For this review, take the finished solid that the model builds, in its own axes (mm). Coordinates: 2 decimals unless noted, no trailing zeros. Loops run counter-clockwise (first coordinate to the right, second up) from the corner with the lowest first, then second, coordinate; pieces in that order, holes last. Notation, with made-up numbers: (-10, -14) -> (41, -14) arc R31 ccw to (41, 24) -> close; hole circle Ø11 at (35, -23). An arc over 180 degrees is marked (long way). One line per item, written item: value.
from build123d import *

# Parameters (mm, degrees)
SALIENTE_EXTRUIR1_DEPTH = 0.25
CORTAR_EXTRUIR1_REACH   = 2.25
CROQUIS2_W              = 0.5
CROQUIS2_H              = 0.2


with BuildPart() as part:
    # Croquis1 → Saliente-Extruir1 (new body)
    with BuildSketch(Plane.XY):
        with BuildLine():
            Line((-0.5, -2.449489743), (-0.5, -3))
            ThreePointArc((-0.5, -3), (0, -3.5), (0.5, -3))
            Line((0.5, -3), (0.5, -2.449489743))
            ThreePointArc((0.5, -2.449489743), (2.5, 0), (0.5, 2.449489743))
            Line((0.5, 2.449489743), (0.5, 6))
            ThreePointArc((0.5, 6), (0, 6.5), (-0.5, 6))
            Line((-0.5, 6), (-0.5, 2.449489743))
            ThreePointArc((-0.5, 2.449489743), (-2.5, 0), (-0.5, -2.449489743))
        make_face()
        with BuildLine():
            ThreePointArc((-2.110242877, -0.25), (-1.411448724, -1.588533128), (0, -2.125))
            ThreePointArc((0, -2.125), (1.411448724, -1.588533128), (2.110242877, -0.25))
            ThreePointArc((2.110242877, -0.25), (1.588533128, 1.411448724), (0, 2.125))
            ThreePointArc((0, 2.125), (-1.588533128, 1.411448724), (-2.110242877, -0.25))
        make_face(mode=Mode.SUBTRACT)
    extrude(amount=SALIENTE_EXTRUIR1_DEPTH)

    # Croquis2 → Cortar-Extruir1 (cut, up to next)
    with BuildSketch(Plane(origin=(0, 0, 0), x_dir=(-1, 0, 0), z_dir=(0, 0, -1)), mode=Mode.PRIVATE) as cortar_extruir1_sk1:
        with Locations((0, 4.4)):
            Rectangle(CROQUIS2_W, CROQUIS2_H)
    cortar_extruir1_tool1 = extrude(cortar_extruir1_sk1.sketch, amount=-CORTAR_EXTRUIR1_REACH, mode=Mode.PRIVATE) & part.part
    add(cortar_extruir1_tool1.solids().sort_by_distance((0, 4.4, 0))[0], mode=Mode.SUBTRACT)
    # Croquis2 → Cortar-Extruir1 (cut, up to next)
    with BuildSketch(Plane(origin=(0, 0, 0), x_dir=(-1, 0, 0), z_dir=(0, 0, -1)), mode=Mode.PRIVATE) as cortar_extruir1_sk2:
        with Locations((0, 4.1)):
            Rectangle(CROQUIS2_W, CROQUIS2_H)
    cortar_extruir1_tool2 = extrude(cortar_extruir1_sk2.sketch, amount=-CORTAR_EXTRUIR1_REACH, mode=Mode.PRIVATE) & part.part
    add(cortar_extruir1_tool2.solids().sort_by_distance((0, 4.1, 0))[0], mode=Mode.SUBTRACT)


solid = part.part
1. Insertion check: pin 1 Ø3 at (x, y) = (-2, -0.5) entering from -Z. The pin has a flat end and moves straight along its axis. Give the tip position at first contact, or say it passes through.
Return value:
pin 1: stops at z = 0
2. Take a section at B-B, the plane y = 0.5. Give the boundary of the cut face in (x, z).
Return value:
outline: (-2.45, 0) -> (-2.07, 0) -> (-2.07, 0.25) -> (-2.45, 0.25) -> close; (2.07, 0) -> (2.45, 0) -> (2.45, 0.25) -> (2.07, 0.25) -> close
3. To check wall thickness, follow probe 1 along Y at (x, z) = (-0.6, 0.2); probe 2 along X at (y, z) = (6, 0.2); probe 3 along Y at (x, z) = (0.55, 0.2). State the ranges of each line that lie inside material, in increasing order. Write a range as from..to.
Return value:
probe 1: y = -2.43..-2.04, 2.04..2.43
probe 2: x = -0.5..0.5
probe 3: y = -2.44..-2.05, 2.05..2.44
4. Take a section at A-A, the plane z = 0.15. Give the boundary of the cut face in (x, y) (3 decimals).
Return value:
outline: (-0.5, -3) arc R0.5 ccw to (0.5, -3) -> (0.5, -2.449) arc R2.5 ccw to (0.5, 2.449) -> (0.5, 6) arc R0.5 ccw to (-0.5, 6) -> (-0.5, 2.449) arc R2.5 ccw to (-0.5, -2.449) -> close; hole circle Ø4.25 at (0, 0); hole (-0.25, 4) -> (0.25, 4) -> (0.25, 4.2) -> (-0.25, 4.2) -> close; hole (-0.25, 4.3) -> (0.25, 4.3) -> (0.25, 4.5) -> (-0.25, 4.5) -> close
5. Take a section at D-D, the plane y = 3.75. Give the boundary of the cut face in (x, z).
Return value:
outline: (-0.5, 0) -> (0.5, 0) -> (0.5, 0.25) -> (-0.5, 0.25) -> close
6. Take a section at C-C, the plane x = -0.35. Give the boundary of the cut face in (y, z).
Return value:
outline: (-3.36, 0) -> (-2.1, 0) -> (-2.1, 0.25) -> (-3.36, 0.25) -> close; (2.1, 0) -> (6.36, 0) -> (6.36, 0.25) -> (2.1, 0.25) -> close
